from build123d import *

# Parameters (mm, degrees)
F1_DEPTH = 25


with BuildPart() as f1:
    # F0 (on Top) → F1 (new body)
    with BuildSketch(Plane.XY):
        with BuildLine():
            Line((-20.7364413533, -16.5), (0, -16.5))
            Line((0, -16.5), (20.7364413533, -16.5))
            ThreePointArc((20.7364413533, -16.5), (25.0176507277, -8.7388301316), (26.5, 0))
            ThreePointArc((26.5, 0), (25.181622021, 8.2544480367), (21.3576669894, 15.6875766379))
            ThreePointArc((21.3576669894, 15.6875766379), (0, 26.5), (-21.3576669894, 15.6875766379))
            ThreePointArc((-21.3576669894, 15.6875766379), (-26.4950658, -0.5113592207), (-20.7364413533, -16.5))
        make_face()
        with BuildLine():
            ThreePointArc((0, -16.5), (-11.6672618896, 11.6672618896), (16.5, 0))
            ThreePointArc((16.5, 0), (11.6672618896, -11.6672618896), (0, -16.5))
        make_face(mode=Mode.SUBTRACT)
        with BuildLine():
            Line((20.7364413533, -16.5), (0, -16.5))
            Line((0, -16.5), (0, -26.5))
            ThreePointArc((0, -26.5), (11.5108644332, -23.8694365246), (20.7364413533, -16.5))
        make_face()
        with BuildLine():
            Line((0, -26.5), (0, -16.5))
            Line((0, -16.5), (-20.7364413533, -16.5))
            ThreePointArc((-20.7364413533, -16.5), (-11.5108644332, -23.8694365246), (0, -26.5))
        make_face()
        with BuildLine():
            Line((45, -16.5), (20.7364413533, -16.5))
            ThreePointArc((20.7364413533, -16.5), (11.5108644332, -23.8694365246), (0, -26.5))
            Line((0, -26.5), (45, -26.5))
            Line((45, -26.5), (45, -16.5))
        make_face()
        with BuildLine():
            ThreePointArc((26.5, 0), (25.0176507277, -8.7388301316), (20.7364413533, -16.5))
            Line((20.7364413533, -16.5), (45, -16.5))
            Line((45, -16.5), (21.3576669894, 15.6875766379))
            ThreePointArc((21.3576669894, 15.6875766379), (25.181622021, 8.2544480367), (26.5, 0))
        make_face()
        with BuildLine():
            Line((-45, -26.5), (0, -26.5))
            ThreePointArc((0, -26.5), (-11.5108644332, -23.8694365246), (-20.7364413533, -16.5))
            Line((-20.7364413533, -16.5), (-45, -16.5))
            Line((-45, -16.5), (-45, -26.5))
        make_face()
        with BuildLine():
            Line((-45, -16.5), (-20.7364413533, -16.5))
            ThreePointArc((-20.7364413533, -16.5), (-26.4950658, -0.5113592207), (-21.3576669894, 15.6875766379))
            Line((-21.3576669894, 15.6875766379), (-45, -16.5))
        make_face()
    extrude(amount=F1_DEPTH)


solid = f1.part
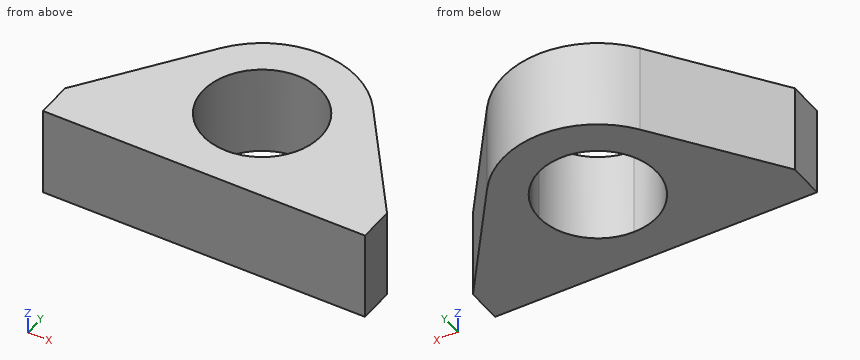
Model file for the job. Use its own axes, mm. Round coordinates to 2 decimals unless told otherwise and drop trailing zeros. Order: outer loops, then holes, each group sorted by start corner. A loop starts at its lowest first (then second) coordinate and runs counter-clockwise, first axis right, second up. Notation, with made-up numbers: M -31.5,-3 L -20.5,-3 A19 ccw -20.5,22 Z; hole C 74.25,55.5 d3. An arc over 180 degrees is marked long. Write each question's results on one line, items separated by ' | '. Start each with the question number.
(1) Saw through at B-B, the plane z = 17.75. Give the cut face in (x, y).
(2) Saw through at D-D, the plane y = 20. Give the cut face in (x, z), then the cut area to 3 significant figures.
(3) Saw through at C-C, the plane x = -3. Give the cut face in (y, z), then the cut area to 3 significant figures.
(4) Saw through at A-A, the plane y = -14. Give the cut face in (x, z), then the cut area to 3 significant figures.
(5) Drop flat-ended pins along their axis: pin 1 (3 mm diameter, centred on x = -4.5, z = 8.5, fed in from +Y); pin 2 (10 mm diameter, centred on x = -32, z = 13.5, fed in from +Y); pin 3 (12 mm diameter, centred on y = -1.5, z = 18, fed in from +X). Give the stop position or say it passes through.
(6) Probe probe 1 along Y at (x, z) = (0, 8); probe 2 along Y at (x, z) = (-1.5, 8); probe 3 along X at (y, z) = (12, 7.75). List the from-to ranges inside material, lowest first. Write a range as from..to.
Established:
1) outline: M -45,-26.5 L 45,-26.5 L 45,-16.5 L 21.36,15.69 A26.5 ccw -21.36,15.69 L -45,-16.5 Z; hole C 0,0 d33
2) outline: M -17.39,0 L 17.39,0 L 17.39,25 L -17.39,25 Z | area: 869 mm^2
3) outline: M -26.5,0 L -16.22,0 L -16.22,25 L -26.5,25 Z; M 16.22,0 L 26.33,0 L 26.33,25 L 16.22,25 Z | area: 509 mm^2
4) outline: M -43.16,0 L -8.73,0 L -8.73,25 L -43.16,25 Z; M 8.73,0 L 43.16,0 L 43.16,25 L 8.73,25 Z | area: 1,720 mm^2
5) pin 1: stops at y = 26.33 | pin 2: stops at y = 8.01 | pin 3: stops at x = 38.39
6) probe 1: y = -26.5..-16.5, 16.5..26.5 | probe 2: y = -26.5..-16.43, 16.43..26.46 | probe 3: x = -24.07..-11.32, 11.32..24.07
